Check sheet for the modelled part. Datum: model origin and axes. Units: mm. Face numbers are marked on the shaded views. A direction names the side the tool comes from. Round coordinates to 2 decimals unless told otherwise and drop trailing zeros. Loops run counter-clockwise (first coordinate to the right, second up) from the corner with the lowest first, then second, coordinate; pieces in that order, holes last. Notation, with made-up numbers: (-15.5, 38.25) - (36.5, 38.25) arc R32 cw to (36.5, 71.25) - close; hole circle Ø6 at (52, 31.25). An arc over 180 degrees is marked (long way). Put each result on its own line as item: value.
Autodesk Inventor part; units mm, degrees
ref_plane "YZ Plane" through (0, 0, 0) normal (1, 0, 0) x (0, 1, 0)
ref_plane "XZ Plane" through (0, 0, 0) normal (0, 1, 0) x (-1, 0, 0)
ref_plane "XY Plane" through (0, 0, 0) normal (0, 0, 1) x (1, 0, 0)
sketch "Esquisse1" plane through (0, 0, 0) normal (0, 1, 0) x (-1, 0, 0)
  circle A0 centre (0, 0) radius 3
  dimension "d0" = 6
extrude "Extrusion1" add sketch "Esquisse1" along normal blind 60
sketch "Esquisse2" plane through (0, 0, 0) normal (0, -1, 0) x (1, 0, 0)
  circle A0 centre (0, 0) radius 3
  circle A1 centre (0, 0) radius 5
  dimension "d3" = 10
extrude "Extrusion2" add sketch "Esquisse2" along normal blind 2 contours A0 | A1
fillet "Congé1" radius 2 1 edges at (-5, -2, 0)
properties part number "vis_6mm_100mm"
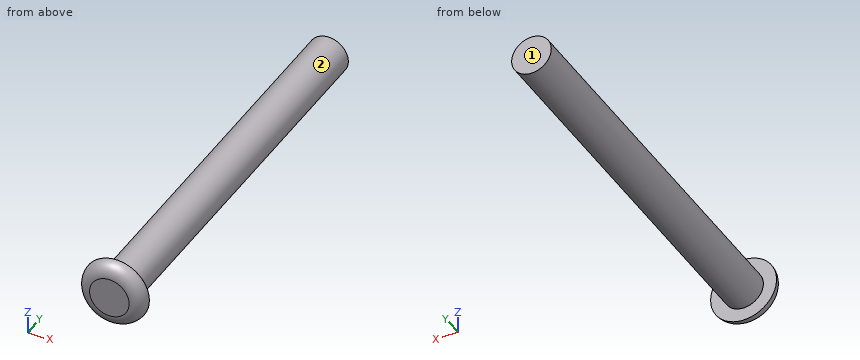
Item 1: Tool access check on the marked faces 1 and 2. Record the directions out of +Z, -Z, +X, -X, +Y, -Y that give a thin tool (end or side, any length) a straight path to the whole face; none if there is none.
Filled sheet:
face 1: +Z, -Z, +X, -X, +Y
face 2: +Y
Item 2: Thickness scan on line 1 (Z direction, x = 0, y = 57); line 2 (Z direction, x = -2.75, y = 22); line 3 (Y direction, x = 3.25, z = 3.25). Record the ranges inside material, lowest first. Write a range as from..to.
Filled sheet:
line 1: -3..3
line 2: -1.2..1.2
line 3: -1.21..0
Item 3: Go/stop test with flat-tipped pins: pin 1 (6 mm diameter, centred on x = -4, y = 43, fed in from +Z); pin 2 (2 mm diameter, centred on x = -3, y = 45.5, fed in from -Z); pin 3 (1.5 mm diameter, centred on y = 32, z = -3.5, fed in from +X). Record where each tip stops, or that it passes through.
Filled sheet:
pin 1: z = 2.83
pin 2: z = -2.24
pin 3: x = 1.2
Item 4: Section check C-C on y = 16.5. Enter the section's corners in (x, z).
Filled sheet:
outline: circle Ø6 at (0, 0)
